```python
from build123d import *

# Parameters (mm, degrees)
CYLINDER1760_R               = 9
CYLINDER1760_DEPTH           = 4
CYLINDER1760_PLACEMENT_ANGLE = 225
BOX711_W                     = 28.8
BOX711_H                     = 2
BOX711_DEPTH                 = 4
COMPOUND890_PLACEMENT_ANGLE  = 225
CYLINDER1692_R               = 1.5
CYLINDER1692_DEPTH           = 60
CYLINDER1689_R               = 1.5
CYLINDER1689_DEPTH           = 60
CYLINDER1690_R               = 1.5
CYLINDER1690_DEPTH           = 60
CYLINDER1691_R               = 1.5
CYLINDER1691_DEPTH           = 60
COMPOUND833_PLACEMENT_ANGLE  = 225
CYLINDER1645_R               = 4
CYLINDER1645_DEPTH           = 4
CYLINDER1645_PLACEMENT_ANGLE = 225
BOX657_W                     = 42
BOX657_H                     = 24
BOX657_DEPTH                 = 2
COMPOUND818_PLACEMENT_ANGLE  = 225
CHAMFER058_SIZE              = 2


with BuildPart() as obj1:
    # Cylinder1760 → Cylinder1760 (new body)
    with BuildSketch(Plane.XY):
        Circle(CYLINDER1760_R)
    extrude(amount=CYLINDER1760_DEPTH)


with BuildPart() as obj1_1:
    # Cylinder1760 placement: moved
    add(obj1.part.moved(Location((63.64, -63.64, 64))).rotate(Axis((63.64, -63.64, 64), (0, 0, 1)), CYLINDER1760_PLACEMENT_ANGLE))


with BuildPart() as compound890:
    # Box711 → Box711 (new body)
    with BuildSketch(Plane(origin=(-14.4, 10, 24), x_dir=(1, 0, 0), z_dir=(0, 0, 1))):
        with Locations((14.4, 1)):
            Rectangle(BOX711_W, BOX711_H)
    extrude(amount=BOX711_DEPTH)


with BuildPart() as compound890_1:
    # Compound890 placement: moved
    add(compound890.part.moved(Location((63.64, -63.64, 38))).rotate(Axis((63.64, -63.64, 38), (0, 0, 1)), COMPOUND890_PLACEMENT_ANGLE))


with BuildPart() as obj2:
    # Cylinder1692 → Cylinder1692 (new body)
    with BuildSketch(Plane(origin=(18, 85, -57), x_dir=(1, 0, 0), z_dir=(0, 0, 1))):
        Circle(CYLINDER1692_R)
    extrude(amount=CYLINDER1692_DEPTH)


with BuildPart() as obj3:
    # Cylinder1689 → Cylinder1689 (new body)
    with BuildSketch(Plane(origin=(-18, 85, -57), x_dir=(1, 0, 0), z_dir=(0, 0, 1))):
        Circle(CYLINDER1689_R)
    extrude(amount=CYLINDER1689_DEPTH)


with BuildPart() as obj4:
    # Cylinder1690 → Cylinder1690 (new body)
    with BuildSketch(Plane(origin=(-18, 95, -57), x_dir=(1, 0, 0), z_dir=(0, 0, 1))):
        Circle(CYLINDER1690_R)
    extrude(amount=CYLINDER1690_DEPTH)


with BuildPart() as compound833:
    # Cylinder1691 → Cylinder1691 (new body)
    with BuildSketch(Plane(origin=(18, 95, -57), x_dir=(1, 0, 0), z_dir=(0, 0, 1))):
        Circle(CYLINDER1691_R)
    extrude(amount=CYLINDER1691_DEPTH)

    # Compound833: union obj2, obj3, obj4
    add(obj2.part)
    add(obj3.part)
    add(obj4.part)


with BuildPart() as compound833_1:
    # Compound833 placement: moved
    add(compound833.part.moved(Location((0, 0, 100))).rotate(Axis((0, 0, 100), (0, 0, 1)), COMPOUND833_PLACEMENT_ANGLE))


with BuildPart() as obj5:
    # Cylinder1645 → Cylinder1645 (new body)
    with BuildSketch(Plane.XY):
        Circle(CYLINDER1645_R)
    extrude(amount=CYLINDER1645_DEPTH)


with BuildPart() as obj5_1:
    # Cylinder1645 placement: moved
    add(obj5.part.moved(Location((63.64, -63.64, 76))).rotate(Axis((63.64, -63.64, 76), (0, 0, 1)), CYLINDER1645_PLACEMENT_ANGLE))


with BuildPart() as base_encoder_washer:
    # Box657 → Box657 (new body)
    with BuildSketch(Plane(origin=(-21, -12, 34), x_dir=(1, 0, 0), z_dir=(0, 0, 1))):
        with Locations((21, 12)):
            Rectangle(BOX657_W, BOX657_H)
    extrude(amount=BOX657_DEPTH)


with BuildPart() as base_encoder_washer_1:
    # Compound818 placement: moved
    add(base_encoder_washer.part.moved(Location((63.64, -63.64, 42))).rotate(Axis((63.64, -63.64, 42), (0, 0, 1)), COMPOUND818_PLACEMENT_ANGLE))

    # Cut472: cut obj5
    add(obj5_1.part, mode=Mode.SUBTRACT)


with BuildPart() as base_encoder_washer_2:
    # Cut472 placement: moved
    add(base_encoder_washer_1.part.moved(Location((0, 0, -10))))

    # Cut481: cut Compound833
    add(compound833_1.part, mode=Mode.SUBTRACT)


with BuildPart() as base_encoder_washer_3:
    # Cut481 placement: moved
    add(base_encoder_washer_2.part.moved(Location((0, 0, -3))))

    # Cut522: cut Compound890
    add(compound890_1.part, mode=Mode.SUBTRACT)

    # Cut523: cut obj1
    add(obj1_1.part, mode=Mode.SUBTRACT)

    # Chamfer058
    chamfer058_edges = [base_encoder_washer_3.edges().sort_by_distance(p)[0] for p in [
        (86.974524, -57.276039, 64),
        (57.276039, -86.974524, 64),
    ]]
    chamfer(chamfer058_edges, length=CHAMFER058_SIZE)


solid = base_encoder_washer_3.part
```
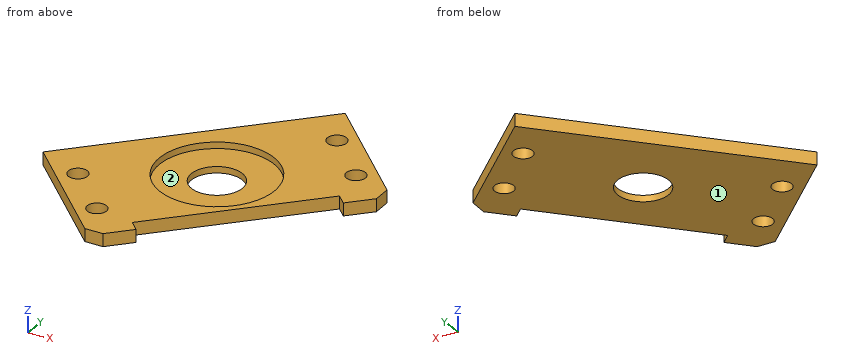
Could you check a few things on this model? Use its own coordinates, in mm. Face numbers are marked on the shaded views. Give positions to 0.01 mm unless a question says otherwise; leave off trailing zeros. Loops run counter-clockwise (first coordinate to the right, second up) from the corner with the lowest first, then second, coordinate; pieces in that order, holes last. Notation, with made-up numbers: (25, 81.25) - (79, 81.25) arc R12 cw to (79, 99.25) - close; hole circle Ø6 at (63, 17.5). An arc over 180 degrees is marked (long way). Answer in a Markdown table with one row per item. Add a question column.
Q1. For pin 1 (2 mm diameter, centred on x = 78.5, y = -63.5, fed in from +Z); pin 2 (5.5 mm diameter, centred on x = 65, y = -64, fed in from +Z), each with a flat end and sliding along its axis, tell me the tip position at first contact or that it passes through.
Q2. We'd pull the mould along X, two halves only. Please class the marked faces 1 and 2: +X half, -X half, draft (parallel to the pull), parting line (faces both ways), or undercut.
Q3. If we section it at D-D (y = -68.5): List the corners of the cut face in (x, z) for me, plus the area to 3 significant figures.
Q4. If we section it at B-B (y = -46.5): List the corners of the cut face in (x, z) for me.
Q5. Please list where these lines run through material, in increasing order: L1, parallel to Y at x = 61.5, z = 64.05; L2, parallel to Y at x = 63.64, z = 63.65; L3, parallel to Y at x = 65, z = 63.8. Write a range as from..to.
Q6. If we section it at C-C (z = 63.55): List the corners of the cut face in (x, y) for me.
Q7. If we section it at A-A (x = 63.64): List the corners of the cut face in (y, z) for me, plus the area to 3 significant figures.
The answers:
| question | item | result |
|---|---|---|
| 1 | pin 1 | stops at z = 65 |
| 1 | pin 2 | stops at z = 64 |
| 2 | face 1 | draft |
| 2 | face 2 | undercut |
| 3 | outline | (41.81, 63) - (72.92, 63) - (72.92, 65) - (71.21, 65) - (71.21, 64) - (56.07, 64) - (56.07, 65) - (41.81, 65) - close |
| 3 | area | 47.1 mm^2 |
| 4 | outline | (63.81, 63) - (71.61, 63) - (71.61, 65) - (63.81, 65) - close; (74.05, 63) - (76.2, 63) - (76.2, 65) - (74.05, 65) - close |
| 5 | L1 | y = -82.75..-81.86, -79.92..-72.38, -54.9..-48.81 |
| 5 | L2 | y = -77.78..-67.64, -59.64..-46.67 |
| 5 | L3 | y = -76.42..-67.4, -59.88..-45.31 |
| 6 | outline | (40.31, -70) - (55.86, -85.56) - (58.69, -85.56) - (61.94, -82.31) - (60.53, -80.89) - (80.89, -60.53) - (82.31, -61.94) - (85.56, -58.69) - (85.56, -55.86) - (70, -40.31) - close; hole circle Ø3 at (47.38, -72.83); hole circle Ø3 at (54.45, -79.9); hole circle Ø8 at (63.64, -63.64); hole circle Ø3 at (72.83, -47.38); hole circle Ø3 at (79.9, -54.45) |
| 7 | outline | (-77.78, 63) - (-67.64, 63) - (-67.64, 64) - (-72.64, 64) - (-72.64, 65) - (-77.78, 65) - close; (-59.64, 63) - (-46.67, 63) - (-46.67, 65) - (-54.64, 65) - (-54.64, 64) - (-59.64, 64) - close |
| 7 | area | 36.2 mm^2 |
